Build history of the part. All positions in model axes, mm. Give positions to 0.01 mm unless a question says otherwise; leave off trailing zeros. Loops run counter-clockwise (first coordinate to the right, second up) from the corner with the lowest first, then second, coordinate; pieces in that order, holes last. Notation, with made-up numbers: M -10,1 L 27,1 A15 cw 27,17 Z; hole C 37.5,79.25 d5. An arc over 180 degrees is marked long. Put each result on its own line as item: value.
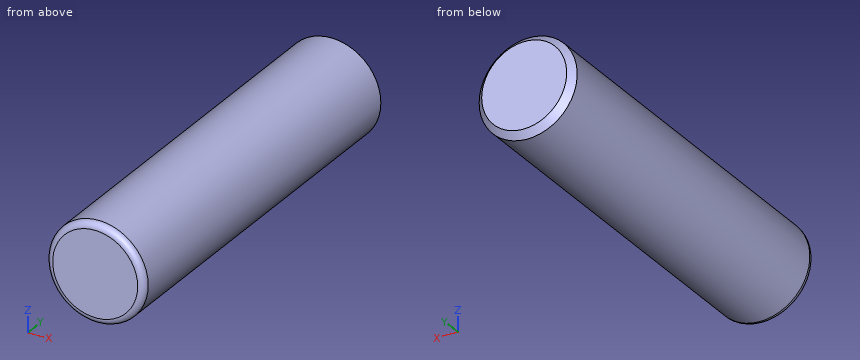
```python
from build123d import *

# Parameters (mm, degrees)
F0_R     = 38.1
F1_DEPTH = 152.4
F2_R     = 5.08
F3_SIZE  = 5.08


with BuildPart() as f1:
    # F0 (on Front) → F1 (new body, symmetric)
    with BuildSketch(Plane.XZ):
        Circle(F0_R)
    extrude(amount=F1_DEPTH, both=True)

    # F2
    f2_edges = [f1.edges().sort_by_distance(p)[0] for p in [
        (-38.1, -152.4, 0),
    ]]
    fillet(f2_edges, radius=F2_R)

    # F3
    f3_edges = [f1.edges().sort_by_distance(p)[0] for p in [
        (38.1, 2.54, 0),
        (-38.1, -147.32, 0),
        (-38.1, 152.4, 0),
    ]]
    chamfer(f3_edges, length=F3_SIZE)


solid = f1.part
```
Q1. Slice it at A-A (y = 61.5). List the corners of the cut face in (x, z), and give its area (3 significant figures).
Here are the results:
outline: C 0,0 d76.2
area: 4,560 mm²
Q2. Probe line 1 (X direction, y = 131, z = -22); line 2 (Z direction, x = -27.5, y = 100); line 3 (Z direction, x = 12.5, y = 49). List the from-to ranges inside material, lowest first. Write a range as from..to.
Here are the results:
line 1: -31.11..31.11
line 2: -26.37..26.37
line 3: -35.99..35.99
Q3. Drop flat-ended pins along their axis: pin 1 Ø3 at (y, z) = (36, 1.5) entering from -X; pin 2 Ø2 at (x, y) = (-17, -18) entering from -Z; pin 3 Ø8 at (x, y) = (-24.5, 53) entering from -Z; pin 4 Ø10 at (y, z) = (-78.5, 10) entering from +X. Give the stop position or say it passes through.
Here are the results:
pin 1: x = -38.1
pin 2: z = -34.58
pin 3: z = -32.11
pin 4: x = 37.77
